Design review of the part built by this model. Coordinates are the model's own, in mm. Round coordinates to 2 decimals unless told otherwise and drop trailing zeros. Write each loop counter-clockwise with the first axis right and the second up, starting at its lowest first coordinate (ties: lowest second). Pieces come first, ordered by that corner, then holes. Notation, with made-up numbers: M 74.5,-35 L 88.5,-35 A29 cw 88.5,3 Z; hole C 32.25,71.5 d5. An arc over 180 degrees is marked long. Use CSV: the item, a comma, the result in double quotes.
from build123d import *

# Parameters (mm, degrees)
SKETCH2_R           = 4.05
BOSS_EXTRUDE1_DEPTH = 1.5


with BuildPart() as part:
    # Sketch2 → Boss-Extrude1 (new body)
    with BuildSketch(Plane.XY):
        with BuildLine():
            Line((-1.5, 5.809475019), (-1.5, 59.037116847))
            add(Edge.make_bspline(
                [(0, 65.809475019), (-1.051472953, 62.487162114), (-1.5, 59.037116847)],
                knots=[0, 0, 0, 1, 1, 1], degree=2))
            add(Edge.make_bspline(
                [(0, 65.809475019), (1.051472953, 62.487162114), (1.5, 59.037116847)],
                knots=[0, 0, 0, 1, 1, 1], degree=2))
            Line((1.5, 59.037116847), (1.5, 5.809475019))
            ThreePointArc((1.5, 5.809475019), (0, -6), (-1.5, 5.809475019))
        make_face()
        Circle(SKETCH2_R, mode=Mode.SUBTRACT)
    extrude(amount=BOSS_EXTRUDE1_DEPTH)


solid = part.part
1) Wall thickness on line 1 along X through (y, z) = (47.5, 0.2); line 2 along Y through (x, z) = (2.5, 1.15); line 3 along Y through (x, z) = (-3, 1.35): over which ranges is each line inside the solid? List them lowest first. Write a range as [from, to].
Answers:
line 1,"[-1.5, 1.5]"
line 2,"[-5.45, -3.19], [3.19, 5.45]"
line 3,"[-5.2, -2.72], [2.72, 5.2]"
2) Add section C-C on y = 38. Write out the cut boundary in (x, z), then the cut area to 3 significant figures.
Answers:
outline,"M -1.5,0 L 1.5,0 L 1.5,1.5 L -1.5,1.5 Z"
area,"4.50 mm²"
3) Add section A-A on y = 0. Write out the cut boundary in (x, z), then the cut area to 3 significant figures.
Answers:
outline,"M -6,0 L -4.05,0 L -4.05,1.5 L -6,1.5 Z; M 4.05,0 L 6,0 L 6,1.5 L 4.05,1.5 Z"
area,"5.85 mm²"
4) For pin 1 Ø5 at (x, y) = (0, 0) entering from -Z, flat-tipped, find the tip position at first contact; note if it passes through.
Answers:
pin 1,"through"
5) Add section B-B on x = -3. Write out the cut boundary in (y, z).
Answers:
outline,"M -5.2,0 L -2.72,0 L -2.72,1.5 L -5.2,1.5 Z; M 2.72,0 L 5.2,0 L 5.2,1.5 L 2.72,1.5 Z"
6) Add section D-D on x = 4.75. Write out the cut boundary in (y, z), then the cut area to 3 significant figures.
Answers:
outline,"M -3.67,0 L 3.67,0 L 3.67,1.5 L -3.67,1.5 Z"
area,"11.0 mm²"
7) The part is to be moulded in two halves that separate along X. For faces 1 (the face through (0, 25, 1.5)), 2 (the face through (-1.5, 32, 1)), 3 (the face through (-0.878, -3.954, 0.74)), 4 (the face through (1.5, 33, 1)), say which applies: released by +X, released by -X, zero draft, split by the parting line, or undercut.
Answers:
face 1,"zero draft"
face 2,"released by -X"
face 3,"undercut"
face 4,"released by +X"
